Verification items for the finished model (mm, model axes). A direction names the side the tool comes from. Coordinates: 2 decimals unless noted, no trailing zeros. Order: outer loops, then holes, each group sorted by start corner. A loop starts at its lowest first (then second) coordinate and runs counter-clockwise, first axis right, second up. Notation, with made-up numbers: M -27,83.25 L -13,83.25 A13 ccw -13,104.25 Z; hole C 69,68 d9. An arc over 180 degrees is marked long. Return JSON: item names as keys, results as strings. Group by question number.
1. Section check B-B, the plane x = 43.5. Record the cut outline in (y, z).
2. Section check A-A, the plane z = 6.75. Record the cut outline in (x, y).
3. Section check D-D, the plane x = 0. Record the cut outline in (y, z), plus the area to 3 significant figures.
4. Mould release check, pull along Y, two halves, no side actions. Record for faces 4 (the flat face through (-28, -25.15, 1)), 5 (the flat face through (48.5, 0, 1)), 6 (the cylindrical face through (40.503, -20.018, 5.465)): +Y half, -Y half, draft (parallel to the pull), parting line (faces both ways), or undercut.
5. Section check C-C, the plane y = -20.15. Record the cut outline in (x, z), plus the area to 3 significant figures.
6. Material ranges on line 1 along Y through (x, z) = (0, 1.25); line 2 along Y through (x, z) = (-43.5, 5.5); line 3 along X through (y, z) = (-20, 1.75), recorded low to high.
7. Gauge pin test, flat ends, axial feed: pin 1 (1 mm diameter, centred on y = -26, z = 1.5, fed in from -X); pin 2 (2.5 mm diameter, centred on x = 43.5, y = -20.15, fed in from +Z); pin 3 (1 mm diameter, centred on y = 26.5, z = 2, fed in from +X); pin 4 (0.9 mm diameter, centred on x = 17.5, z = 1.5, fed in from -Y). Record the tip position at first contact, or that the pin passes through.
8. Set-up check for faces 1 (the flat face through (-1, 0, 3)), 2 (the flat face through (6, 26, 1)), 3 (the flat face through (-27, 25.15, 1)): record each of +Z, -Z, +X, -X, +Y, -Y from which the full face is reachable in a straight line by a thin tool's end or side.
```python
from build123d import *

# Parameters (mm, degrees)
F0_R     = 3
F0_R_2   = 2.2
F0_R_3   = 1.45
F1_DEPTH = 3
F2_DEPTH = 8
F3_SIZE  = 1.5


with BuildPart() as f1:
    # F0 (on Top) → F1 (new body)
    with BuildSketch(Plane.XY):
        with BuildLine():
            Line((48.5, -25.15), (48.5, 25.15))
            Line((48.5, 25.15), (6, 25.15))
            Line((6, 25.15), (6, 27.15))
            ThreePointArc((6, 27.15), (0, 33.15), (-6, 27.15))
            Line((-6, 27.15), (-6, 25.15))
            Line((-6, 25.15), (-48.5, 25.15))
            Line((-48.5, 25.15), (-48.5, -25.15))
            Line((-48.5, -25.15), (-6, -25.15))
            Line((-6, -25.15), (-6, -27.15))
            ThreePointArc((-6, -27.15), (0, -33.15), (6, -27.15))
            Line((6, -27.15), (6, -25.15))
            Line((6, -25.15), (48.5, -25.15))
        make_face()
        with Locations((-43.5, -20.15)):
            Circle(F0_R, mode=Mode.SUBTRACT)
        with Locations((0, -27.15)):
            Circle(F0_R_2, mode=Mode.SUBTRACT)
        with Locations((43.5, -20.15)):
            Circle(F0_R, mode=Mode.SUBTRACT)
        with Locations((-43.5, 20.15)):
            Circle(F0_R, mode=Mode.SUBTRACT)
        with Locations((0, 27.15)):
            Circle(F0_R_2, mode=Mode.SUBTRACT)
        with Locations((43.5, 20.15)):
            Circle(F0_R, mode=Mode.SUBTRACT)
        with Locations((-43.5, 20.15)):
            Circle(F0_R)
        with Locations((-43.5, 20.15)):
            Circle(F0_R_3, mode=Mode.SUBTRACT)
        with Locations((-43.5, -20.15)):
            Circle(F0_R)
        with Locations((-43.5, -20.15)):
            Circle(F0_R_3, mode=Mode.SUBTRACT)
        with Locations((43.5, -20.15)):
            Circle(F0_R)
        with Locations((43.5, -20.15)):
            Circle(F0_R_3, mode=Mode.SUBTRACT)
        with Locations((43.5, 20.15)):
            Circle(F0_R)
        with Locations((43.5, 20.15)):
            Circle(F0_R_3, mode=Mode.SUBTRACT)
    extrude(amount=F1_DEPTH)

    # F0 (on Top) → F2 (join)
    with BuildSketch(Plane.XY):
        with Locations((-43.5, 20.15)):
            Circle(F0_R)
        with Locations((-43.5, 20.15)):
            Circle(F0_R_3, mode=Mode.SUBTRACT)
        with Locations((-43.5, -20.15)):
            Circle(F0_R)
        with Locations((-43.5, -20.15)):
            Circle(F0_R_3, mode=Mode.SUBTRACT)
        with Locations((43.5, 20.15)):
            Circle(F0_R)
        with Locations((43.5, 20.15)):
            Circle(F0_R_3, mode=Mode.SUBTRACT)
        with Locations((43.5, -20.15)):
            Circle(F0_R)
        with Locations((43.5, -20.15)):
            Circle(F0_R_3, mode=Mode.SUBTRACT)
    extrude(amount=F2_DEPTH)

    # F3
    f3_edges = [f1.edges().sort_by_distance(p)[0] for p in [
        (-2.2, 27.15, 3),
        (-2.2, -27.15, 3),
    ]]
    chamfer(f3_edges, length=F3_SIZE)


solid = f1.part
```
Answers follow:
{
 "1": {"outline": "M -25.15,0 L -21.6,0 L -21.6,8 L -23.15,8 L -23.15,3 L -25.15,3 Z; M -18.7,0 L 18.7,0 L 18.7,8 L 17.15,8 L 17.15,3 L -17.15,3 L -17.15,8 L -18.7,8 Z; M 21.6,0 L 25.15,0 L 25.15,3 L 23.15,3 L 23.15,8 L 21.6,8 Z"},
 "2": {"outline": "C -43.5,-20.15 d6; C -43.5,20.15 d6; C 43.5,-20.15 d6; C 43.5,20.15 d6; hole C -43.5,-20.15 d2.9; hole C -43.5,20.15 d2.9; hole C 43.5,-20.15 d2.9; hole C 43.5,20.15 d2.9"},
 "3": {"outline": "M -33.15,0 L -29.35,0 L -29.35,1.5 L -30.85,3 L -33.15,3 Z; M -24.95,0 L 24.95,0 L 24.95,1.5 L 23.45,3 L -23.45,3 L -24.95,1.5 Z; M 29.35,0 L 33.15,0 L 33.15,3 L 30.85,3 L 29.35,1.5 Z", "area": "168 mm^2"},
 "4": {"face 4": "-Y half", "face 5": "draft", "face 6": "undercut"},
 "5": {"outline": "M -48.5,0 L -44.95,0 L -44.95,8 L -46.5,8 L -46.5,3 L -48.5,3 Z; M -42.05,0 L 42.05,0 L 42.05,8 L 40.5,8 L 40.5,3 L -40.5,3 L -40.5,8 L -42.05,8 Z; M 44.95,0 L 48.5,0 L 48.5,3 L 46.5,3 L 46.5,8 L 44.95,8 Z", "area": "305 mm^2"},
 "6": {"line 1": "-33.15 to -29.35, -24.95 to 24.95, 29.35 to 33.15", "line 2": "-23.15 to -21.6, -18.7 to -17.15, 17.15 to 18.7, 21.6 to 23.15", "line 3": "-48.5 to -44.94, -42.06 to 42.06, 44.94 to 48.5"},
 "7": {"pin 1": "x = -6", "pin 2": "through", "pin 3": "x = 6", "pin 4": "y = -25.15"},
 "8": {"face 1": "+Z", "face 2": "+Z, -Z, +X, +Y", "face 3": "+Z, -Z, -X, +Y"}
}
